from build123d import *

# Parameters (mm, degrees)
BOSS_EXTRUDE1_DEPTH     = 1.5875
F_4_CLEARANCE_HOLE1_D   = 3.2639
F_10_CLEARANCE_HOLE1_D  = 5.1054
F_1_4_CLEARANCE_HOLE1_D = 6.5278


with BuildPart() as part:
    # Sketch1 → Boss-Extrude1 (new, symmetric)
    with BuildSketch(Plane(origin=(0, 0, 0), x_dir=(1, 0, 0), z_dir=(0, 1, 0))):
        Polygon((-69.85, -69.85), (-79.375, -69.85), (-79.375, 79.375), (69.85, 79.375), (69.85, 69.85), (69.85, -69.85), align=None)
    extrude(amount=BOSS_EXTRUDE1_DEPTH, both=True)

    # #4 Clearance Hole1 (through all)
    with Locations(Plane(origin=(0, 1.5875, 0), x_dir=(1, 0, 0), z_dir=(0, 1, 0))):
        with Locations((-74.6125, 4.7625), (-74.6125, 39.6875), (-74.6125, 74.6125), (-39.6875, 74.6125), (-4.7625, 74.6125), (-74.6125, -30.1625)):
            Hole(F_4_CLEARANCE_HOLE1_D / 2)

    # #10 Clearance Hole1 (through all)
    with Locations(Plane(origin=(0, 1.5875, 0), x_dir=(1, 0, 0), z_dir=(0, 1, 0))):
        with Locations((-63.5, -60.325), (-63.5, 63.5), (60.325, -19.05), (-22.225, -11.43), (22.225, -11.43)):
            Hole(F_10_CLEARANCE_HOLE1_D / 2)

    # 1/4 Clearance Hole1 (through all)
    with Locations(Plane(origin=(0, 1.5875, 0), x_dir=(1, 0, 0), z_dir=(0, 1, 0))):
        with Locations((-22.225, -11.43), (22.225, -11.43)):
            Hole(F_1_4_CLEARANCE_HOLE1_D / 2)


solid = part.part
The listing builds one solid part. Answer for the finished solid, in the listing's coordinates (mm). Round coordinates to 2 decimals unless told otherwise and drop trailing zeros. Answer in a Markdown table with one row per item. Add a question column.
1) The part is cut by section A-A on z = 11.43. Count the separate pieces of the cut face and the enclosed holes in it, plus the area to 3 significant figures.
2) Determine the mould class of faces 1 (the face through (-6, 0, 69.85)), 2 (the face through (-5.516, -0.022, -73.165)), 3 (the face through (-4, -1.588, -6)), 4 (the face through (-75.49, -0.022, -41.064)) for opening direction Z: pulls with the +Z half, pulls with the -Z half, needs draft (parallel to the pull), parting line crosses it, or undercut.
3) Flat-ended cylindrical pins translate along their axes: pin 1 Ø4 at (x, z) = (-39.69, -74.61) entering from +Y; pin 2 Ø2.5 at (x, z) = (-74.61, 30.16) entering from -Y. Find the tip coordinate at first contact, or state that the pin passes through.
4) Consider line 1 along Z through (x, y) = (-63.5, -0.6) (3 decimals); line 2 along X through (y, z) = (-0.9, 11.43) (3 decimals); line 3 along X through (y, z) = (-0.75, 19.5) (3 decimals). Determine where each line is inside the solid, lowest interval first. Write a range as from..to.
Findings below:
| question | item | result |
|---|---|---|
| 1 | separate pieces | 3 |
| 1 | enclosed holes | 0 |
| 1 | area | 432 mm² |
| 2 | face 1 | pulls with the +Z half |
| 2 | face 2 | undercut |
| 2 | face 3 | needs draft |
| 2 | face 4 | undercut |
| 3 | pin 1 | stops at y = 1.59 |
| 3 | pin 2 | passes through |
| 4 | line 1 | z = -79.375..-66.053, -60.947..57.772, 62.878..69.85 |
| 4 | line 2 | x = -79.375..-25.489, -18.961..18.961, 25.489..69.85 |
| 4 | line 3 | x = -79.375..57.812, 62.838..69.85 |
